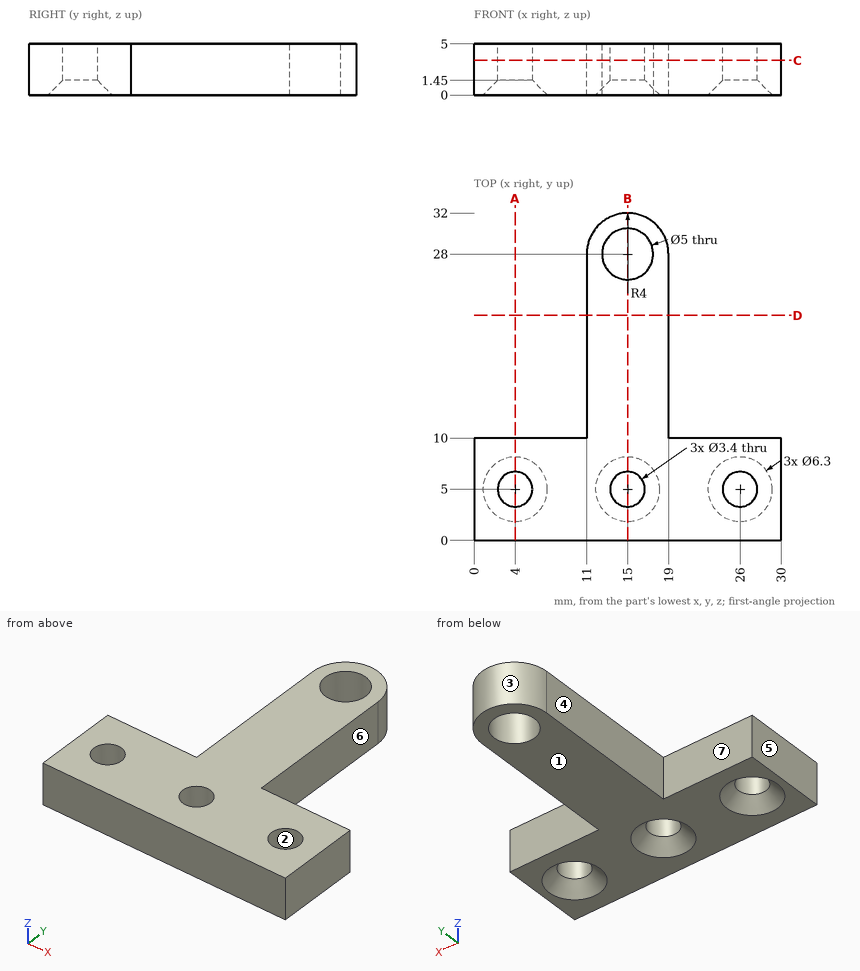
Source: three-view drawing plus pictorial views. Frame: mm from the lowest corner of the part. A direction names the side the tool comes from. Give positions to 0.01 mm unless a question says otherwise; leave off trailing zeros. Loops run counter-clockwise (first coordinate to the right, second up) from the corner with the lowest first, then second, coordinate; pieces in that order, holes last.
1) Section query B-B on x = 15. Return the cut outline in (y, z).
A:
outline: (0, 0) - (1.85, 0) - (3.3, 1.45) - (3.3, 5) - (0, 5) - close; (6.7, 1.45) - (8.15, 0) - (25.5, 0) - (25.5, 5) - (6.7, 5) - close; (30.5, 0) - (32, 0) - (32, 5) - (30.5, 5) - close
2) Reachability of the marked faces 5, 6 and 7 from +Z, -Z, +X, -X, +Y, -Y: full face, straight path, thin tool, end or side. Return the list, or none.
A:
face 5: +Z, -Z, -X, +Y, -Y
face 6: +Z, -Z, +X, +Y
face 7: +Z, -Z, -X, +Y
3) Section query C-C on z = 3.4. Return the cut outline in (x, y), and give its area (3 significant figures).
A:
outline: (0, 0) - (30, 0) - (30, 10) - (19, 10) - (19, 28) arc R4 ccw to (11, 28) - (11, 10) - (0, 10) - close; hole circle Ø3.4 at (4, 5); hole circle Ø5 at (15, 28); hole circle Ø3.4 at (15, 5); hole circle Ø3.4 at (26, 5)
area: 422 mm2
4) Line query: L1, parallel to X at y = 5, z = 2.45; L2, parallel to Y at x = 15, z = 1.5; L3, parallel to Y at x = 13.5, z = 2.55. Output: solid intervals per line, ascending.
A:
L1: x = 0 to 2.3, 5.7 to 13.3, 16.7 to 24.3, 27.7 to 30
L2: y = 0 to 3.3, 6.7 to 25.5, 30.5 to 32
L3: y = 0 to 4.2, 5.8 to 26, 30 to 31.71
5) Mould query, pull axis X, two halves, no side actions, for the marked faces 1, 2, 3 and 4. Classes: released by +X, released by -X, zero draft, split by the parting line, or undercut.
A:
face 1: zero draft
face 2: undercut
face 3: split by the parting line
face 4: released by -X
6) Contact query for flat-ended pins moving along their axis: pin 1 (1.5 mm diameter, centred on y = 21.5, z = 3.5, fed in from +X); pin 2 (1 mm diameter, centred on y = 23, z = 4.5, fed in from -X); pin 3 (12 mm diameter, centred on x = 26.5, y = 11, fed in from -Z); pin 4 (4.5 mm diameter, centred on x = 15, y = 5, fed in from -Z). Output: stop coordinate, or through.
A:
pin 1: stops at x = 19
pin 2: stops at x = 11
pin 3: stops at z = 0
pin 4: stops at z = 0.9
7) Section query A-A on x = 4. Return the cut outline in (y, z).
A:
outline: (0, 0) - (1.85, 0) - (3.3, 1.45) - (3.3, 5) - (0, 5) - close; (6.7, 1.45) - (8.15, 0) - (10, 0) - (10, 5) - (6.7, 5) - close
8) Section query D-D on y = 22. Return the cut outline in (x, z), and give its area (3 significant figures).
A:
outline: (11, 0) - (19, 0) - (19, 5) - (11, 5) - close
area: 40.0 mm2
